The model under review builds one solid part; all positions refer to its coordinate system, in mm. A direction names the side the tool comes from. Give positions to 0.01 mm unless a question says otherwise; leave off trailing zeros. Order: outer loops, then holes, each group sorted by start corner. A loop starts at its lowest first (then second) coordinate and runs counter-clockwise, first axis right, second up. Notation, with made-up numbers: (-17, -16.75) - (38, -16.75) arc R23 cw to (38, 8.25) - close; hole circle Ø11 at (54.25, 68.25). An arc over 180 degrees is marked (long way). Use CSV: the item, a comma, the result in double quotes. Start each with the question number.
1. Take a section at B-B, the plane x = 0. State the section outline as (y, z) points.
2. For pin 1 (6.5 mm diameter, centred on x = 0, y = 10, fed in from -Z), flat-tipped, find the tip position at first contact; note if it passes through.
3. Draft analysis for pull direction X (two halves, no side actions). For faces 4 (the cylindrical face through (0.759, 6.583, 2.958)), 5 (the cylindrical face through (0, 16, 3)), 6 (the flat face through (-6, 5, 3)), state which applies: released by +X, released by -X, zero draft, split by the parting line, or undercut.
4. To check wall thickness, follow line 1 (Y direction, x = 0, z = 2.55); line 2 (Y direction, x = -3, z = 3.8); line 3 (X direction, y = 13, z = 3.65). State the ranges of each line that lie inside material, in increasing order. Write a range as [from, to].
5. Machinability: for faces 1 (the cylindrical face through (-4, -2, 3)), 2 (the cylindrical face through (4, -2, 3)), 3 (the flat face through (6, 5, 3)), which of the approach directions +Z, -Z, +X, -X, +Y, -Y give a long, thin tool a straight path to every point of the face, cutting with its end or side? Answer none if there is none.
6. Take a section at A-A, the plane z = 3. State the section outline as (x, y) points, then the cut area to 3 significant figures.
7. Take a section at D-D, the plane x = -2. State the section outline as (y, z) points, then the cut area to 3 significant figures.
8. Take a section at C-C, the plane y = -2.5. State the section outline as (x, z) points, then the cut area to 3 significant figures.
```python
from build123d import *

# Parameters (mm, degrees)
BOSS_EXTRUDE1_DEPTH       = 6
M8X1_0_TAPPED_HOLE1_D     = 7
M8X1_0_TAPPED_HOLE1_DEPTH = 19
M8X1_0_TAPPED_HOLE1_TIP   = 2.103012167
CUT_EXTRUDE1_DEPTH        = 23.649503306
CUT_EXTRUDE1_DEPTH_BACK   = 5
SKETCH4_W                 = 9.430442817
SKETCH4_H                 = 6.865018404


with BuildPart() as part:
    # Sketch1 → Boss-Extrude1 (new body)
    with BuildSketch(Plane.XY):
        with BuildLine():
            Line((-4, -5), (4, -5))
            Line((4, -5), (4, 0))
            Line((4, 0), (6, 0))
            Line((6, 0), (6, 10))
            ThreePointArc((6, 10), (0, 16), (-6, 10))
            Line((-6, 10), (-6, 0))
            Line((-6, 0), (-4, 0))
            Line((-4, 0), (-4, -5))
        make_face()
    extrude(amount=BOSS_EXTRUDE1_DEPTH)

    # M8x1.0 Tapped Hole1
    with Locations(Plane.XY.offset(6)):
        with Locations((0, 10)):
            Hole(M8X1_0_TAPPED_HOLE1_D / 2, depth=M8X1_0_TAPPED_HOLE1_DEPTH)
            with Locations((0, 0, -(M8X1_0_TAPPED_HOLE1_DEPTH + M8X1_0_TAPPED_HOLE1_TIP / 2))):  # 118° drill point
                Cone(0, M8X1_0_TAPPED_HOLE1_D / 2, M8X1_0_TAPPED_HOLE1_TIP, mode=Mode.SUBTRACT)

    # Sketch4 → Cut-Extrude1 (cut, two sides: drawn at the far end of the back side and taken through both)
    with BuildSketch(Plane.XZ.offset(5).offset(-CUT_EXTRUDE1_DEPTH_BACK)):
        with Locations((0.112084889, 2.942713281)):
            Rectangle(SKETCH4_W, SKETCH4_H)
        with BuildLine():
            Line((-1, 6), (1, 6))
            ThreePointArc((1, 6), (4, 3), (1, 0))
            Line((1, 0), (-1, 0))
            ThreePointArc((-1, 0), (-4, 3), (-1, 6))
        make_face(mode=Mode.SUBTRACT)
    extrude(amount=CUT_EXTRUDE1_DEPTH + CUT_EXTRUDE1_DEPTH_BACK, mode=Mode.SUBTRACT)


solid = part.part
```
Determined:
1,outline,"(-5, 0) - (6.5, 0) - (6.5, 6) - (-5, 6) - close; (13.5, 0) - (16, 0) - (16, 6) - (13.5, 6) - close"
2,pin 1,"passes through"
3,face 4,"undercut"
3,face 5,"split by the parting line"
3,face 6,"released by -X"
4,line 1,"y = [-5, 6.5], [13.5, 16]"
4,line 2,"y = [-5, 8.2], [11.8, 15.2]"
4,line 3,"x = [-5.2, -1.8], [1.8, 5.2]"
5,face 1,"-X, -Y"
5,face 2,"+X, -Y"
5,face 3,"+Z, -Z, +X, +Y, -Y"
6,outline,"(-6, 0) - (-4, 0) - (-4, -5) - (4, -5) - (4, 0) - (6, 0) - (6, 10) arc R6 ccw to (-6, 10) - close; hole circle Ø7 at (0, 10)"
6,area,"178 mm²"
7,outline,"(-5, 0.17) - (0, 0.17) - (0, 0) - (7.13, 0) - (7.13, 6) - (0, 6) - (0, 5.83) - (-5, 5.83) - close; (12.87, 0) - (15.66, 0) - (15.66, 6) - (12.87, 6) - close"
7,area,"87.8 mm²"
8,outline,"(-1, 0) - (1, 0) arc R3 ccw to (1, 6) - (-1, 6) arc R3 ccw to start"
8,area,"40.3 mm²"
